```python
from build123d import *

# Parameters (mm, degrees)
ESQUISSE2_W                 = 150
ESQUISSE2_H                 = 26
T_LE_DE_BASE_PLI_E1_DEPTH   = 4
PLI_START                   = -13
PLI_ESQUISS_1_DEPTH         = 26
PLI_ESQUISS_1_2_DEPTH       = 26
ESQUISSE9_R                 = 2.5
ESQUISSE9_R_2               = 1.25
BOSS_EXTRU_1_DEPTH          = 1.5
ENL_V_START                 = -4
ENL_V_MAT_EXTRU_1_OUTLINE_R = 1.25
ENL_V_MAT_EXTRU_1_DEPTH     = 4
ESQUISSE11_W                = 4
ESQUISSE11_H                = 26
BOSS_EXTRU_2_DEPTH          = 40
BOSS_EXTRU_3_DEPTH          = 4
ESQUISSE12_R                = 2
ENL_V_MAT_EXTRU_5_DEPTH     = 151.86574353
ENL_V_MAT_EXTRU_6_REACH     = 152.866
ESQUISSE12_4_R              = 3.5
ESQUISSE12_4_R_2            = 2


# Read off the part's stored shape, not the designer's step: Pli esquissé1, Enlèv. mat.-Extru.1
# Sheet-metal steps are written as plain solids
with BuildPart() as part:
    # Esquisse2 → Tôle de base pliée1 (new body)
    with BuildSketch(Plane(origin=(0, 0, 0), x_dir=(1, 0, 0), z_dir=(0, 1, 0))):
        Rectangle(ESQUISSE2_W, ESQUISSE2_H)
    extrude(amount=-T_LE_DE_BASE_PLI_E1_DEPTH)

    # Pli esquissé1 outline → Pli esquissé1 (cut)
    with BuildSketch(Plane.XY.offset(PLI_START)):
        with BuildLine():
            Line((75, 0), (56.347473252, 0))
            Line((56.347473252, 0), (46.142385808, -3.714348068))
            ThreePointArc((46.142385808, -3.714348068), (45.344875155, -3.928040403), (44.522373197, -4))
            Line((44.522373197, -4), (75, -4))
            Line((75, -4), (75, 0))
        make_face()
    extrude(amount=PLI_ESQUISS_1_DEPTH, mode=Mode.SUBTRACT)

    # Pli esquiss_1 2 outline → Pli esquiss_1 2 (add)
    with BuildSketch(Plane.XY.offset(PLI_START)):
        with BuildLine():
            Line((56.347473252, 0), (73.884342049, 6.382898245))
            Line((73.884342049, 6.382898245), (72.516261476, 10.141668728))
            Line((72.516261476, 10.141668728), (44.774305234, 0.044422416))
            ThreePointArc((44.774305234, 0.044422416), (44.650282444, 0.011190609), (44.522373197, 0))
            Line((44.522373197, 0), (56.347473252, 0))
        make_face()
    extrude(amount=PLI_ESQUISS_1_2_DEPTH)

    # Esquisse9 → Boss.-Extru.1 (add)
    # profile 1 of 4: a face of its own
    with BuildSketch(Plane(origin=(5.223321668, -14.350958338, 0), x_dir=(0.9396926207859082, 0.34202014332566943, 0), z_dir=(-0.34202014332566943, 0.9396926207859082, 0))):
        with Locations(Location((55.111650787, 10.5, 0), (0, 0, 90))):
            Circle(ESQUISSE9_R)
        with Locations(Location((55.111650787, 10.5, 0), (0, 0, 180))):
            Circle(ESQUISSE9_R_2, mode=Mode.SUBTRACT)
    # profile 2 of 4: a face of its own
    with BuildSketch(Plane(origin=(5.223321668, -14.350958338, 0), x_dir=(0.9396926207859082, 0.34202014332566943, 0), z_dir=(-0.34202014332566943, 0.9396926207859082, 0))):
        with Locations(Location((68.611650787, 10.5, 0), (0, 0, 90))):
            Circle(ESQUISSE9_R)
        with Locations(Location((68.611650787, 10.5, 0), (0, 0, 180))):
            Circle(ESQUISSE9_R_2, mode=Mode.SUBTRACT)
    # profile 3 of 4: a face of its own
    with BuildSketch(Plane(origin=(5.223321668, -14.350958338, 0), x_dir=(0.9396926207859082, 0.34202014332566943, 0), z_dir=(-0.34202014332566943, 0.9396926207859082, 0))):
        with Locations((68.611650787, -10.5)):
            Circle(ESQUISSE9_R)
        with Locations((68.611650787, -10.5)):
            Circle(ESQUISSE9_R_2, mode=Mode.SUBTRACT)
    # profile 4 of 4: a face of its own
    with BuildSketch(Plane(origin=(5.223321668, -14.350958338, 0), x_dir=(0.9396926207859082, 0.34202014332566943, 0), z_dir=(-0.34202014332566943, 0.9396926207859082, 0))):
        with Locations((55.111650787, -10.5)):
            Circle(ESQUISSE9_R)
        with Locations((55.111650787, -10.5)):
            Circle(ESQUISSE9_R_2, mode=Mode.SUBTRACT)
    extrude(amount=BOSS_EXTRU_1_DEPTH)

    # Enlèv. mat.-Extru.1 outline → Enlèv. mat.-Extru.1 (cut)
    with BuildSketch(Plane(origin=(5.223321668, -14.350958338, 0), x_dir=(0.9396926207859082, 0.34202014332566943, 0), z_dir=(-0.34202014332566943, 0.9396926207859082, 0)).offset(ENL_V_START)):
        with Locations((68.611650787, 10.5)):
            Circle(ENL_V_MAT_EXTRU_1_OUTLINE_R)
        with Locations((68.611650787, -10.5)):
            Circle(ENL_V_MAT_EXTRU_1_OUTLINE_R)
        with Locations((55.111650787, 10.5)):
            Circle(ENL_V_MAT_EXTRU_1_OUTLINE_R)
        with Locations((55.111650787, -10.5)):
            Circle(ENL_V_MAT_EXTRU_1_OUTLINE_R)
    extrude(amount=ENL_V_MAT_EXTRU_1_DEPTH, mode=Mode.SUBTRACT)

    # Esquisse11 → Boss.-Extru.2 (add)
    with BuildSketch(Plane(origin=(0, 0, 0), x_dir=(1, 0, 0), z_dir=(0, 1, 0))):
        with Locations((-73, 0)):
            Rectangle(ESQUISSE11_W, ESQUISSE11_H)
    extrude(amount=BOSS_EXTRU_2_DEPTH)

    # Esquisse3D1 → Boss.-Extru.3 (add, along a direction that is not the sketch's normal)
    with BuildSketch(Plane(origin=(-71, 40, -13), x_dir=(0.7710162866859277, -0.533933827949873, 0.34705698816741753), z_dir=(0.5693204883585811, 0.8221156740600114, 0))):
        Polygon((0, 0), (9.023481692, -24.38394509), (74.915650416, 0), (65.892168724, 24.38394509), align=None)
    extrude(amount=-BOSS_EXTRU_3_DEPTH, dir=(0, 1, 0))

    # Esquisse12 → Enlèv. mat.-Extru.5 (cut, through all)
    with BuildSketch(Plane(origin=(-71, 0, 0), x_dir=(0, 0, -1), z_dir=(1, 0, 0))):
        with Locations((-3, 7)):
            Circle(ESQUISSE12_R)
        with Locations((0, 17)):
            Circle(ESQUISSE12_R)
    extrude(amount=-ENL_V_MAT_EXTRU_5_DEPTH, mode=Mode.SUBTRACT)

    # Enlèv. mat.-Extru.6: up to this plane
    enl_v_mat_extru_6_end = Plane(origin=(-4.291041229, -6.196390829, 0), z_dir=(0.5693204883585812, 0.8221156740600113, 0))
    # Esquisse12<4> → Enlèv. mat.-Extru.6 (cut, up to the surface)
    with BuildSketch(Plane(origin=(-71, 0, 0), x_dir=(0, 0, -1), z_dir=(1, 0, 0)), mode=Mode.PRIVATE) as enl_v_mat_extru_6_sk1:
        with Locations(Location((-3, 7, 0), (0, 0, 90))):
            Circle(ESQUISSE12_4_R)
        with Locations((-3, 7)):
            Circle(ESQUISSE12_4_R_2, mode=Mode.SUBTRACT)
    enl_v_mat_extru_6_tool1 = split(extrude(enl_v_mat_extru_6_sk1.sketch, amount=ENL_V_MAT_EXTRU_6_REACH, mode=Mode.PRIVATE), bisect_by=enl_v_mat_extru_6_end, keep=Keep.BOTH, mode=Mode.PRIVATE)
    add(enl_v_mat_extru_6_tool1.solids().sort_by_distance((-71, 3.598995, 3))[0], mode=Mode.SUBTRACT)
    # Esquisse12<4> → Enlèv. mat.-Extru.6 (cut, up to the surface)
    with BuildSketch(Plane(origin=(-71, 0, 0), x_dir=(0, 0, -1), z_dir=(1, 0, 0)), mode=Mode.PRIVATE) as enl_v_mat_extru_6_sk2:
        with Locations((-3, 7)):
            Circle(ESQUISSE12_4_R_2)
    enl_v_mat_extru_6_tool2 = split(extrude(enl_v_mat_extru_6_sk2.sketch, amount=ENL_V_MAT_EXTRU_6_REACH, mode=Mode.PRIVATE), bisect_by=enl_v_mat_extru_6_end, keep=Keep.BOTH, mode=Mode.PRIVATE)
    add(enl_v_mat_extru_6_tool2.solids().sort_by_distance((-71, 7, 3))[0], mode=Mode.SUBTRACT)
    # Esquisse12<4> → Enlèv. mat.-Extru.6 (cut, up to the surface)
    with BuildSketch(Plane(origin=(-71, 0, 0), x_dir=(0, 0, -1), z_dir=(1, 0, 0)), mode=Mode.PRIVATE) as enl_v_mat_extru_6_sk3:
        with Locations(Location((0, 17, 0), (0, 0, 90))):
            Circle(ESQUISSE12_4_R)
        with Locations((0, 17)):
            Circle(ESQUISSE12_4_R_2, mode=Mode.SUBTRACT)
    enl_v_mat_extru_6_tool3 = split(extrude(enl_v_mat_extru_6_sk3.sketch, amount=ENL_V_MAT_EXTRU_6_REACH, mode=Mode.PRIVATE), bisect_by=enl_v_mat_extru_6_end, keep=Keep.BOTH, mode=Mode.PRIVATE)
    add(enl_v_mat_extru_6_tool3.solids().sort_by_distance((-71, 13.598995, 0))[0], mode=Mode.SUBTRACT)
    # Esquisse12<4> → Enlèv. mat.-Extru.6 (cut, up to the surface)
    with BuildSketch(Plane(origin=(-71, 0, 0), x_dir=(0, 0, -1), z_dir=(1, 0, 0)), mode=Mode.PRIVATE) as enl_v_mat_extru_6_sk4:
        with Locations((0, 17)):
            Circle(ESQUISSE12_4_R_2)
    enl_v_mat_extru_6_tool4 = split(extrude(enl_v_mat_extru_6_sk4.sketch, amount=ENL_V_MAT_EXTRU_6_REACH, mode=Mode.PRIVATE), bisect_by=enl_v_mat_extru_6_end, keep=Keep.BOTH, mode=Mode.PRIVATE)
    add(enl_v_mat_extru_6_tool4.solids().sort_by_distance((-71, 17, 0))[0], mode=Mode.SUBTRACT)


solid = part.part
```
For this review, take the finished solid that the model builds, in its own axes (mm). A direction names the side the tool comes from. Round coordinates to 2 decimals unless told otherwise and drop trailing zeros. Write each loop counter-clockwise with the first axis right and the second up, starting at its lowest first coordinate (ties: lowest second). Pieces come first, ordered by that corner, then holes. Notation, with made-up numbers: M -24,40.5 L 6,40.5 A20 ccw 6,44.5 Z; hole C -36,48 d4. An arc over 180 degrees is marked long. One line per item, written item: value. Start each with the question number.
(1) We need section A-A (z = -5.5). Give the boundary of the cut face in (x, y), and give its area (3 significant figures).
(2) The part is to be moulded in two halves that separate along Y. For faces 1 (the flat face through (-73, 40, 0)), 2 (the cylindrical face through (67.58, 9.13, 12.02)), 3 (the flat face through (-20, 4, -13)), say which applies: released by +Y, released by -Y, zero draft, split by the parting line, or undercut.
(3) We need section B-B (y = 17). Give the boundary of the cut face in (x, z), and give its area (3 significant figures).
(4) Wall thickness on line 1 (Z direction, x = -43.5, y = 17); line 2 (Y direction, x = 42.5, z = -0.75); line 3 (X direction, y = 19.5, z = 0.25): over which ranges is each line inside the solid? List them lowest first.
(5) Insertion check: pin 1 (2.5 mm diameter, centred on y = 17, z = 0, fed in from -X) (3 decimals); pin 2 (4 mm diameter, centred on x = -55, z = 7.5, fed in from +Y); pin 3 (6 mm diameter, centred on x = -38.5, z = -5.5, fed in from +Y); pin 4 (3.5 mm diameter, centred on y = 7, z = 3, fed in from +X). Each pin has a flat end and moves straight along its axis. Give the tip position at first contact, or say it passes through.
(6) We need section C-C (x = -58). Give the boundary of the cut face in (y, z).
(7) Machinability: for faces 4 (the cylindrical face through (-73, 9, 3)), 5 (the flat face through (15, 0, 0)), 6 (the flat face through (-45, 0, 0)), which of the approach directions +Z, -Z, +X, -X, +Y, -Y give a long, thin tool a straight path to every point of the face, cutting with its end or side? Answer none if there is none.
(8) We need section D-D (x = 32.5). Give the boundary of the cut face in (y, z), and give its area (3 significant figures).
Result:
1. outline: M -75,-4 L 44.52,-4 A4.74 ccw 46.14,-3.71 L 73.88,6.38 L 72.52,10.14 L 44.77,0.04 A0.74 cw 44.52,0 L -13.24,0 L -71,40 L -75,40 Z; hole M -71,0 L -19.01,0 L -71,36 Z
1. area: 979 mm²
2. face 1: released by +Y
2. face 2: undercut
2. face 3: zero draft
3. outline: M -75,-13 L -71,-13 L -71,-2 L -75,-2 Z; M -75,2 L -71,2 L -71,13 L -75,13 Z; M -43.56,-13 L -37.79,-13 L -37.79,-3.5 L -43.56,-3.5 Z; M -43.56,3.5 L -37.79,3.5 L -37.79,13 L -43.56,13 Z
3. area: 198 mm²
4. line 1: -13 to -3.5, 3.5 to 13
4. line 2: -4 to 0
4. line 3: -75 to -71
5. pin 1: through
5. pin 2: y = 30.3
5. pin 3: y = 19.57
5. pin 4: x = 73.88
6. outline: M -4,-13 L 0,-13 L 0,13 L -4,13 Z; M 27,-13 L 31,-13 L 31,13 L 27,13 Z
7. face 4: -X
7. face 5: +Z, -Z, +Y
7. face 6: +Z, -Z
8. outline: M -4,-13 L 0,-13 L 0,13 L -4,13 Z
8. area: 104 mm²
